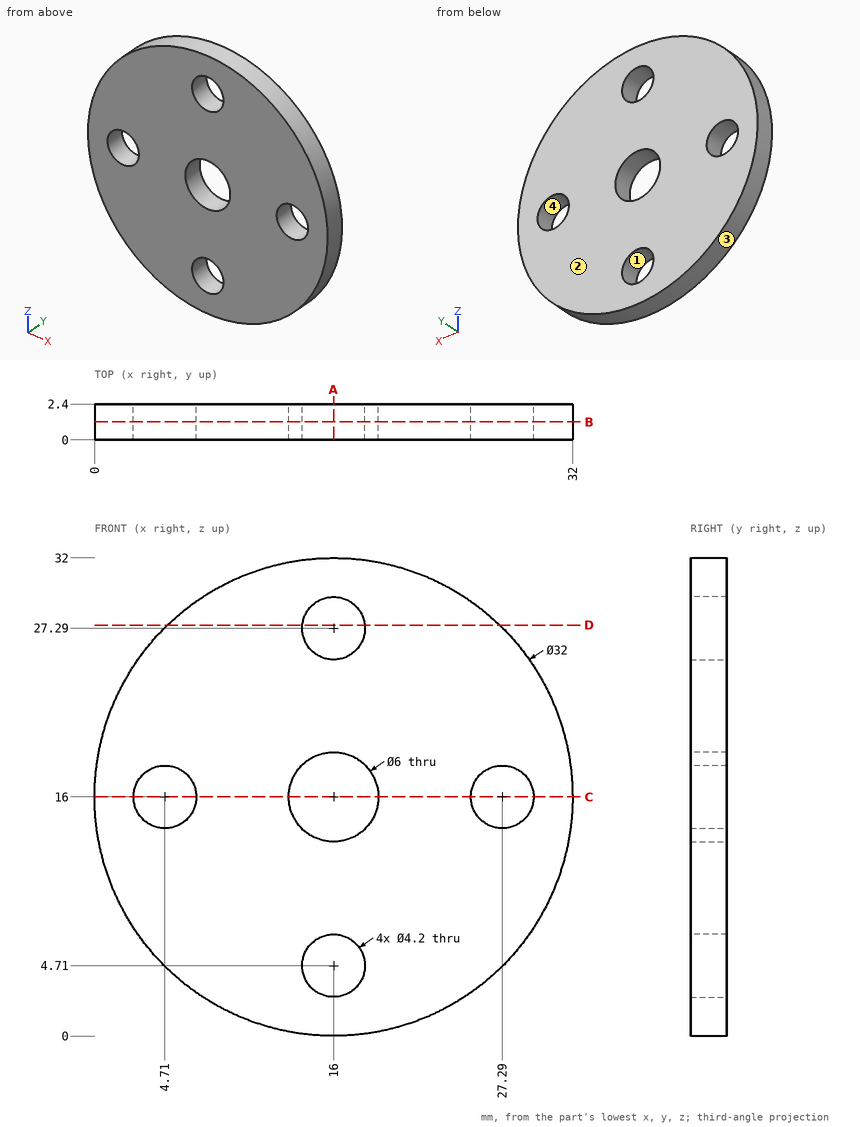
Input: dimensioned drawing with shaded views. Units: mm. Origin: part minimum x, y, z. Give positions to 0.01 mm unless a question says otherwise; leave off trailing zeros. Loops run counter-clockwise (first coordinate to the right, second up) from the corner with the lowest first, then second, coordinate; pieces in that order, holes last. Notation, with made-up numbers: (32, -16.5) - (55, -16.5) arc R22 ccw to (55, 5.5) - close; hole circle Ø3 at (-39.75, 27.5). An arc over 180 degrees is marked (long way). Answer as CSV lines item,"result". Start each with the question number.
(1) Pin query (flat end, axial travel): P1, Ø6, axis at x = 6.5, z = 23.5, coming from the -Y side; P2, Ø2.5, axis at x = 4.71, z = 16, coming from the +Y side. Return the tip coordinate at first contact, or that it passes through.
(2) Section query B-B (y = 1.2). Output: boundary loops of the cut face in (x, z).
(3) Ray query, line 1 along X through (y, z) = (1.45, 16); line 2 along X through (y, z) = (0.45, 27); line 3 along X through (y, z) = (1.25, 27.29). Return the intervals inside material, ascending. Write a range as [from, to].
(4) Mould query, pull axis X, two halves, no side actions, for the marked faces 1, 2, 3 and 4. Classes: +X half, -X half, draft (parallel to the pull), parting line (faces both ways), or undercut.
(5) Section query D-D (z = 27.5). Output: boundary loops of the cut face in (x, y).
(6) Section query A-A (x = 16). Output: boundary loops of the cut face in (y, z), and give its area (3 significant figures).
(7) Section query C-C (z = 16). Output: boundary loops of the cut face in (x, y).
Worked answers:
1,P1,"stops at y = 0"
1,P2,"passes through"
2,outline,"circle Ø32 at (16, 16); hole circle Ø4.2 at (4.71, 16); hole circle Ø6 at (16, 16); hole circle Ø4.2 at (16, 4.71); hole circle Ø4.2 at (16, 27.29); hole circle Ø4.2 at (27.29, 16)"
3,line 1,"x = [0, 2.61], [6.81, 13], [19, 25.19], [29.39, 32]"
3,line 2,"x = [4.38, 13.92], [18.08, 27.62]"
3,line 3,"x = [4.66, 13.9], [18.1, 27.34]"
4,face 1,"undercut"
4,face 2,"draft"
4,face 3,"parting line"
4,face 4,"undercut"
5,outline,"(4.88, 0) - (13.91, 0) - (13.91, 2.4) - (4.88, 2.4) - close; (18.09, 0) - (27.12, 0) - (27.12, 2.4) - (18.09, 2.4) - close"
6,outline,"(0, 0) - (2.4, 0) - (2.4, 2.61) - (0, 2.61) - close; (0, 6.81) - (2.4, 6.81) - (2.4, 13) - (0, 13) - close; (0, 19) - (2.4, 19) - (2.4, 25.19) - (0, 25.19) - close; (0, 29.39) - (2.4, 29.39) - (2.4, 32) - (0, 32) - close"
6,area,"42.2 mm^2"
7,outline,"(0, 0) - (2.61, 0) - (2.61, 2.4) - (0, 2.4) - close; (6.81, 0) - (13, 0) - (13, 2.4) - (6.81, 2.4) - close; (19, 0) - (25.19, 0) - (25.19, 2.4) - (19, 2.4) - close; (29.39, 0) - (32, 0) - (32, 2.4) - (29.39, 2.4) - close"
